Study the drawing (mm; zero at the part's minimum x, y, z) and answer. A direction names the side the tool comes from. Round coordinates to 2 decimals unless told otherwise and drop trailing zeros. Write each loop counter-clockwise with the first axis right and the second up, starting at its lowest first coordinate (ties: lowest second). Pieces come first, ordered by that corner, then holes.
(1) For the marked faces 1, 2 and 3, determine the directions among +Z, -Z, +X, -X, +Y, -Y from which every point of the face is accessible in a straight line to the end or side of a thin tool.
(2) A cutting plane is placed at A-A, the plane y = 3. Give the vertices of the cut face in (x, z), and give its area (3 significant figures).
(3) Each of these flat-tipped pins is pushed along its axis until it touches: pin 1 Ø3 at (y, z) = (2, 14.5) entering from -X; pin 2 Ø1.5 at (y, z) = (4, 34.5) entering from +X; pin 3 Ø0.6 at (x, y) = (12, 3.5) entering from +Z. Where does it stop, or does it pass through?
(4) Find the intervals of material crossed by probe 1 along Y at (x, z) = (8.5, 2.8); probe 2 along X at (y, z) = (4.1, 25.1); probe 3 along Z at (x, y) = (8.5, 3.3), in increasing order.
(5) A cutting plane is placed at D-D, the plane z = 7. Give the vertices of the cut face in (x, y).
(6) A cutting plane is placed at C-C, the plane z = 25.1. Give the vertices of the cut face in (x, y), and give its area (3 significant figures).
(7) The mould has two halves that part along X. Classify the marked faces 4, 5 and 6: +X half, -X half, draft (parallel to the pull), parting line (faces both ways), or undercut.
(8) A cutting plane is placed at B-B, the plane x = 8.5. Give the vertices of the cut face in (y, z).
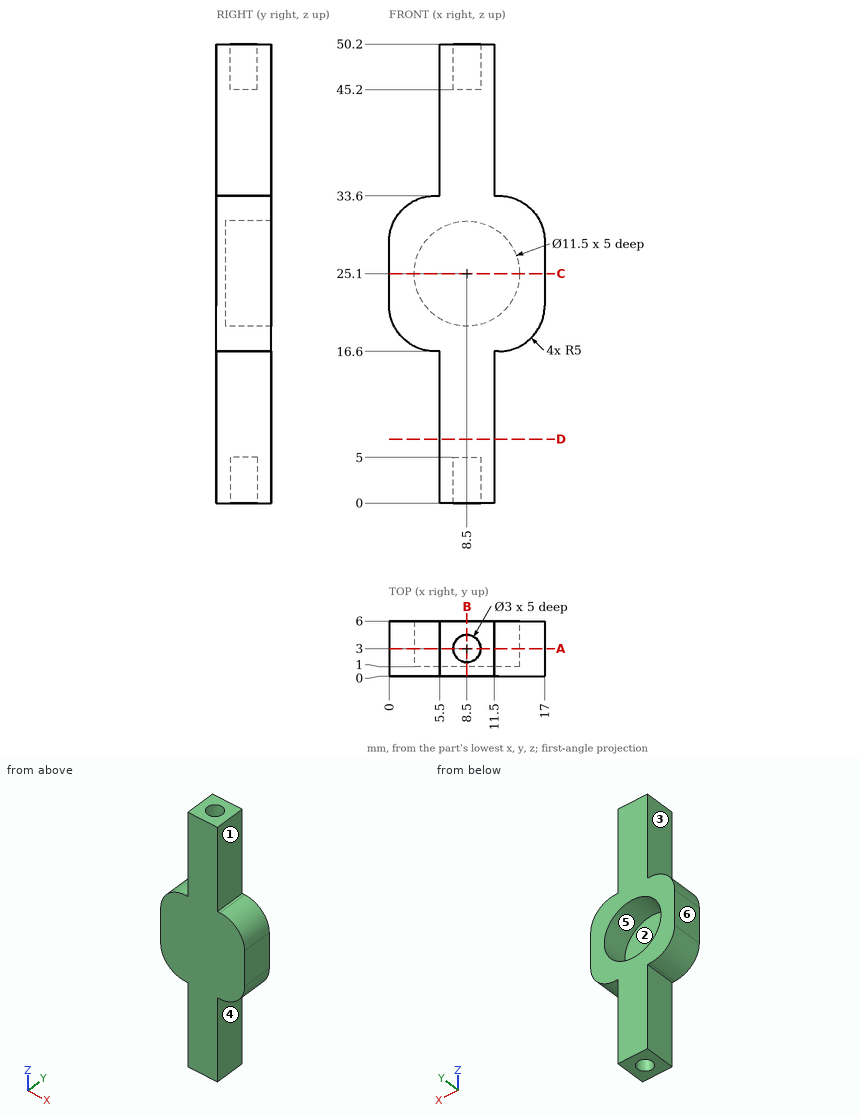
Solutions:
1. face 1: +Z, +X, +Y, -Y
1. face 2: +Y
1. face 3: +Z, -X, +Y, -Y
2. outline: (0, 21.6) arc R5 ccw to (5, 16.6) - (5.5, 16.6) - (5.5, 0) - (7, 0) - (7, 5) - (10, 5) - (10, 0) - (11.5, 0) - (11.5, 16.6) - (12, 16.6) arc R5 ccw to (17, 21.6) - (17, 28.6) arc R5 ccw to (12, 33.6) - (11.5, 33.6) - (11.5, 50.2) - (10, 50.2) - (10, 45.2) - (7, 45.2) - (7, 50.2) - (5.5, 50.2) - (5.5, 33.6) - (5, 33.6) arc R5 ccw to (0, 28.6) - close; hole circle Ø11.5 at (8.5, 25.1)
2. area: 333 mm2
3. pin 1: stops at x = 5.5
3. pin 2: stops at x = 11.5
3. pin 3: stops at z = 33.6
4. probe 1: y = 0 to 1.5, 4.5 to 6
4. probe 2: x = 0 to 2.75, 14.25 to 17
4. probe 3: z = 5 to 19.35, 30.85 to 45.2
5. outline: (5.5, 0) - (11.5, 0) - (11.5, 6) - (5.5, 6) - close
6. outline: (0, 0) - (17, 0) - (17, 6) - (14.25, 6) - (14.25, 1) - (2.75, 1) - (2.75, 6) - (0, 6) - close
6. area: 44.5 mm2
7. face 4: +X half
7. face 5: undercut
7. face 6: -X half
8. outline: (0, 0) - (1.5, 0) - (1.5, 5) - (4.5, 5) - (4.5, 0) - (6, 0) - (6, 19.35) - (1, 19.35) - (1, 30.85) - (6, 30.85) - (6, 50.2) - (4.5, 50.2) - (4.5, 45.2) - (1.5, 45.2) - (1.5, 50.2) - (0, 50.2) - close
